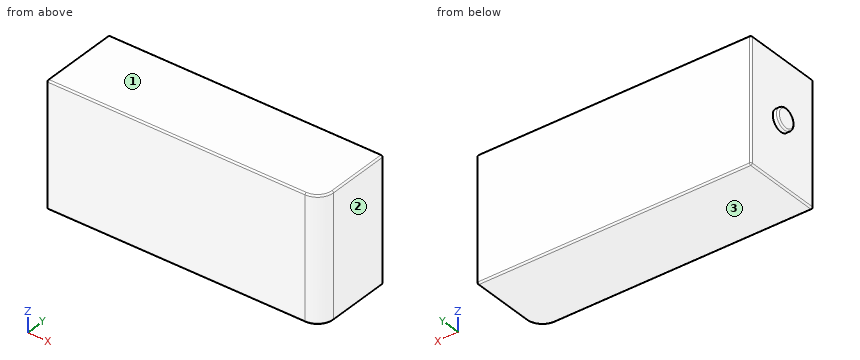
from build123d import *

# Parameters (mm, degrees)
F0_W     = 51.54
F0_H     = 23.2
F1_DEPTH = 15.06
F2_R     = 1.97
F3_DEPTH = 1
F4_R     = 0.3
F5_R     = 3
F6_R     = 0.3


with BuildPart() as f1:
    # F0 (on Front) → F1 (new body)
    with BuildSketch(Plane.XZ):
        Rectangle(F0_W, F0_H)
    extrude(amount=F1_DEPTH)

    # F2 (on face) → F3 (join)
    with BuildSketch(Plane(origin=(-25.77, 0, 0), x_dir=(0, -1, 0), z_dir=(-1, 0, 0))):
        with Locations((7.203062, 0)):
            Circle(F2_R)
    extrude(amount=F3_DEPTH)

    # F4
    f4_edges = [f1.edges().sort_by_distance(p)[0] for p in [
        (-26.77, -5.233062, 0),
    ]]
    fillet(f4_edges, radius=F4_R)

    # F5
    f5_edges = [f1.edges().sort_by_distance(p)[0] for p in [
        (25.77, -15.06, 0),
    ]]
    fillet(f5_edges, radius=F5_R)

    # F6
    f6_edges = [f1.edges().sort_by_distance(p)[0] for p in [
        (-1.5, -15.06, -11.6),
        (-1.5, -15.06, 11.6),
        (-25.77, -15.06, 0),
        (-25.77, -7.53, -11.6),
        (-25.77, 0, 0),
        (-25.77, -7.53, 11.6),
        (0, 0, -11.6),
        (0, 0, 11.6),
        (25.77, 0, 0),
    ]]
    fillet(f6_edges, radius=F6_R)


solid = f1.part
Design review of the part built by this model. Coordinates are the model's own, in mm. Face numbers are marked on the shaded views. Coordinates: 2 decimals unless noted, no trailing zeros. Loops run counter-clockwise (first coordinate to the right, second up) from the corner with the lowest first, then second, coordinate; pieces in that order, holes last. Notation, with made-up numbers: M 31.5,21.25 L 78.5,21.25 A24 ccw 78.5,54.25 Z; hole C 55.5,-22.75 d7. An arc over 180 degrees is marked long. Answer as CSV lines item,"result".
Item 1: Add section B-B on z = 3.25. State the section outline as (x, y) points.
Answer list:
outline,"M -25.77,-14.76 A0.3 ccw -25.47,-15.06 L 22.77,-15.06 A3 ccw 25.77,-12.06 L 25.77,-0.3 A0.3 ccw 25.47,0 L -25.47,0 A0.3 ccw -25.77,-0.3 Z"
Item 2: For probe 1 along X at (y, z) = (-7.5, -4.75); probe 2 along X at (y, z) = (-13.5, -8.5), list the stretches that pass through material, from the lowest coordinate up.
Answer list:
probe 1,"-25.77 to 25.77"
probe 2,"-25.77 to 25.4"
Item 3: The part is to be moulded in two halves that separate along Z. For the marked faces 1, 2 and 3, say which applies: pulls with the +Z half, pulls with the -Z half, needs draft (parallel to the pull), parting line crosses it, or undercut.
Answer list:
face 1,"pulls with the +Z half"
face 2,"needs draft"
face 3,"pulls with the -Z half"
Item 4: Add section C-C on z = 0. State the section outline as (x, y) points, plus the area to 3 significant figures.
Answer list:
outline,"M -26.77,-8.87 A0.3 ccw -26.47,-9.17 L -25.77,-9.17 L -25.77,-14.76 A0.3 ccw -25.47,-15.06 L 22.77,-15.06 A3 ccw 25.77,-12.06 L 25.77,-0.3 A0.3 ccw 25.47,0 L -25.47,0 A0.3 ccw -25.77,-0.3 L -25.77,-5.23 L -26.47,-5.23 A0.3 ccw -26.77,-5.53 Z"
area,"778 mm²"
Item 5: Add section A-A on y = -1.75. State the section outline as (x, z) points, plus the area to 3 significant figures.
Answer list:
outline,"M -25.77,-11.3 A0.3 ccw -25.47,-11.6 L 25.47,-11.6 A0.3 ccw 25.77,-11.3 L 25.77,11.3 A0.3 ccw 25.47,11.6 L -25.47,11.6 A0.3 ccw -25.77,11.3 Z"
area,"1,200 mm²"
Item 6: For P1, Ø1, axis at y = -5.5, z = -3.5, coming from the -X side, flat-tipped, find the tip position at first contact; note if it passes through.
Answer list:
P1,"x = -25.77"
